Here's how the part is built. I have some questions about the finished solid (model axes, mm). A direction names the side the tool comes from. Coordinates: 2 decimals unless noted, no trailing zeros. Loops run counter-clockwise (first coordinate to the right, second up) from the corner with the lowest first, then second, coordinate; pieces in that order, holes last. Notation, with made-up numbers: (35.25, -7) -> (41.25, -7) arc R22 cw to (41.25, 11) -> close; hole circle Ø11 at (-3, -23.5). An arc over 180 degrees is marked (long way). Answer as a JSON object with one key per item and string values. Group by question number.
Q1. I want a section at B-B on y = -47.25. Write out the boundary of the cut face in (x, z), then the cut area to 3 significant figures.
Q2. Thinking about a two-plate mould opening in X: for faces 1 (the flat face through (-15.333, -48, 2)), 2 (the flat face through (-16, -48, 2)), 3 (the flat face through (16, -48, 2)), 4 (the flat face through (11, -48, 2.8)), which applies, released by +X, released by -X, zero draft, split by the parting line, or undercut?
Q3. On a 3-axis mill with a long thin cutter (end or side, diameter ignored), from which of +Z, -Z, +X, -X, +Y, -Y can I reach the whole of each face in a straight line? I mean faces 5 (the flat face through (5.333, -48, 2)), 6 (the flat face through (-26, -48, 2)). Say none if no direction works.
Q4. I want a section at A-A on z = 2.2. Write out the boundary of the cut face in (x, y).
Q5. I need wall thicknesses on line 1 (X direction, y = -53.25, z = 2.3). Which ranges of the line are inside material? Lowest first, please.
```python
from build123d import *

# Parameters (mm, degrees)
SKETCH021_W            = 10
SKETCH021_H            = 13
PAD_DEPTH              = 1.2
PAD_FACE5_W            = 13
PAD_FACE5_H            = 10
PAD008_DEPTH           = 1
PAD008_FACE8_W         = 13
PAD008_FACE8_H         = 1
PAD009_DEPTH           = 32
LINEARPATTERN004_COUNT = 4
LINEARPATTERN004_PITCH = 10.6666666667


with BuildPart() as part:
    # Sketch021 → Pad (new body)
    with BuildSketch(Plane.XY):
        Rectangle(SKETCH021_W, SKETCH021_H)
    pad = extrude(amount=PAD_DEPTH)

    # Pad Face5 → Pad008 (add)
    with BuildSketch(Plane(origin=(0, 0, 0), x_dir=(0, -1, 0), z_dir=(0, 0, -1))):
        Rectangle(PAD_FACE5_W, PAD_FACE5_H)
    extrude(amount=PAD008_DEPTH)

    # Pad008 Face8 → Pad009 (add)
    with BuildSketch(Plane(origin=(5, 0, -0.5), x_dir=(0, -1, 0), z_dir=(1, 0, 0))):
        Rectangle(PAD008_FACE8_W, PAD008_FACE8_H)
    extrude(amount=PAD009_DEPTH)

    # LinearPattern004: Pad ×4
    with Locations(*[(i * LINEARPATTERN004_PITCH, 0, 0) for i in range(1, LINEARPATTERN004_COUNT)]):
        add(pad)


with BuildPart() as part_1:
    # Body004 placement: moved
    add(part.part.moved(Location((-21, -48, 1.6))))


solid = part_1.part
```
Result set:
{
 "1": {"outline": "(-26, 0.6) -> (16, 0.6) -> (16, 2.8) -> (6, 2.8) -> (6, 1.6) -> (5.33, 1.6) -> (5.33, 2.8) -> (-4.67, 2.8) -> (-4.67, 1.6) -> (-5.33, 1.6) -> (-5.33, 2.8) -> (-15.33, 2.8) -> (-15.33, 1.6) -> (-16, 1.6) -> (-16, 2.8) -> (-26, 2.8) -> close", "area": "90.0 mm²"},
 "2": {"face 1": "undercut", "face 2": "undercut", "face 3": "released by +X", "face 4": "zero draft"},
 "3": {"face 5": "+Z, +Y, -Y", "face 6": "+Z, -Z, -X, +Y, -Y"},
 "4": {"outline": "(-26, -54.5) -> (-16, -54.5) -> (-16, -41.5) -> (-26, -41.5) -> close; (-15.33, -54.5) -> (-5.33, -54.5) -> (-5.33, -41.5) -> (-15.33, -41.5) -> close; (-4.67, -54.5) -> (5.33, -54.5) -> (5.33, -41.5) -> (-4.67, -41.5) -> close; (6, -54.5) -> (16, -54.5) -> (16, -41.5) -> (6, -41.5) -> close"},
 "5": {"line 1": "x = -26 to -16, -15.33 to -5.33, -4.67 to 5.33, 6 to 16"}
}
